Answer from the drawing. Dimensions are ordinates in mm from the lowest x, y and z of the part. A direction names the side the tool comes from. Coordinates: 2 decimals unless noted, no trailing zeros. Write each loop counter-clockwise with the first axis right and the second up, starting at its lowest first coordinate (ties: lowest second). Pieces come first, ordered by that corner, then holes.
(1) Section B-B on y = 27.5 is taken. Write down the section's boundary in (x, z), then the cut area to 3 significant figures.
(2) Given pin 1 (1.5 mm diameter, centred on x = 15.5, z = 18, fed in from -Y); pin 2 (21 mm diameter, centred on x = 28.5, y = 19, fed in from -Z); pin 3 (6 mm diameter, centred on x = 22, y = 32, fed in from -Z); pin 4 (8 mm diameter, centred on x = 32, z = 14, fed in from +Y) (1 decimal), each flat-ended and moving along its own axis, determine where each tip first touches the part or whether it passes through.
(3) Which of the six approach directions +Z, -Z, +X, -X, +Y, -Y give full straight-line access (tool end or side, diameter ignored) to the marked faces 4 and 5?
(4) Find the intervals of material crossed by probe 1 along Z at (x, y) = (6.5, 39.5); probe 2 along X at (y, z) = (21.5, 5.25) (1 decimal); probe 3 along X at (y, z) = (35.5, 15.5) (1 decimal), in increasing order.
(5) Section C-C on x = 22.5 is taken. Write down the section's boundary in (y, z), then the cut area to 3 significant figures.
(6) The mould has two halves that part along Y. Classify the marked faces 1, 2 and 3: +Y half, -Y half, draft (parallel to the pull), parting line (faces both ways), or undercut.
(7) Section D-D on z = 7.5 is taken. Write down the section's boundary in (x, y) (1 decimal), then the cut area to 3 significant figures.
(8) Section A-A on z = 20.5 is taken. Write down the section's boundary in (x, y), then the cut area to 3 significant figures.
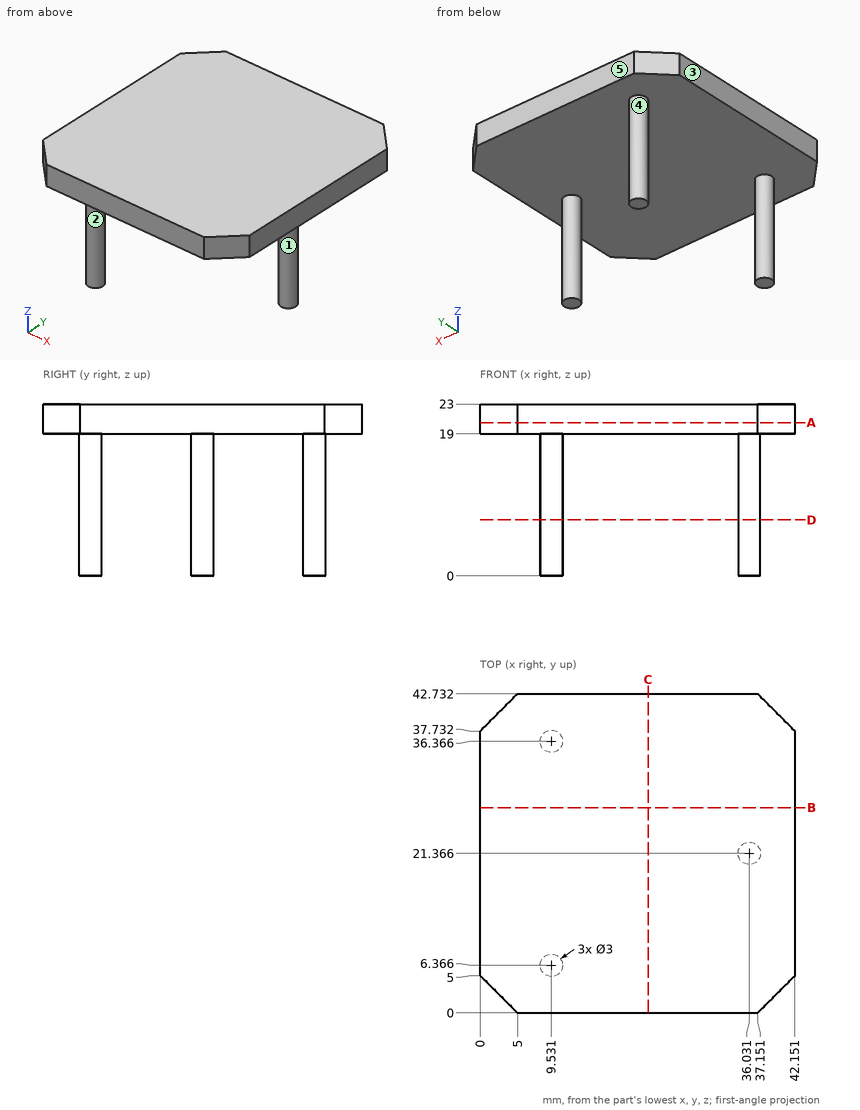
Response:
1. outline: (0, 19) - (42.15, 19) - (42.15, 23) - (0, 23) - close
1. area: 169 mm2
2. pin 1: passes through
2. pin 2: stops at z = 0
2. pin 3: stops at z = 19
2. pin 4: stops at y = 22.9
3. face 4: -Z
3. face 5: +Z, -Z, +X, -X, +Y
4. probe 1: z = 19 to 23
4. probe 2: x = 34.5 to 37.5
4. probe 3: x = 8.3 to 10.8
5. outline: (0, 19) - (42.73, 19) - (42.73, 23) - (0, 23) - close
5. area: 171 mm2
6. face 1: parting line
6. face 2: undercut
6. face 3: draft
7. outline: circle Ø3 at (9.5, 6.4); circle Ø3 at (9.5, 36.4); circle Ø3 at (36, 21.4)
7. area: 21.2 mm2
8. outline: (0, 5) - (5, 0) - (37.15, 0) - (42.15, 5) - (42.15, 37.73) - (37.15, 42.73) - (5, 42.73) - (0, 37.73) - close
8. area: 1,750 mm2
